Check sheet for the modelled part. Datum: model origin and axes. Units: mm. A direction names the side the tool comes from. Round coordinates to 2 decimals unless told otherwise and drop trailing zeros. Order: outer loops, then holes, each group sorted by start corner. A loop starts at its lowest first (then second) coordinate and runs counter-clockwise, first axis right, second up. Notation, with made-up numbers: (54, 35) -> (100, 35) arc R21 cw to (100, 48) -> close; hole circle Ø2 at (48.5, 12). An arc over 180 degrees is marked (long way). Answer in a Markdown table with one row per item.
Autodesk Inventor part; units mm, degrees
ref_plane "YZ Plane" through (0, 0, 0) normal (1, 0, 0) x (0, 1, 0)
ref_plane "XZ Plane" through (0, 0, 0) normal (0, 1, 0) x (-1, 0, 0)
ref_plane "XY Plane" through (0, 0, 0) normal (0, 0, 1) x (1, 0, 0)
sketch "Sketch1" plane through (0, 0, 0) normal (0, 0, 1) x (1, 0, 0)
  line L0 (0, 0) -> (6.15, 0)
  line L1 (6.15, 0) -> (6.15, 4.4)
  line L2 (6.15, 4.4) -> (0, 4.4)
  line L3 (0, 4.4) -> (0, 0)
  dimension "d0" = 6.15
  dimension "d1" = 4.4
extrude "Extrusion1" add sketch "Sketch1" against normal blind 4.7
sketch "Sketch2" plane through (0, 0, -4.7) normal (0, 0, -1) x (-1, 0, 0)
  line L0 (-6.15, 0) -> (-6.15, 4.4)
  line L1 (0, 4.4) -> (0, 0)
  line L2 (-6.15, 4.4) -> (0, 4.4)
  circle A0 centre (-4.545, 3.353) radius 0.25
  circle A1 centre (-1.605, 3.353) radius 0.25
  circle A2 centre (-4.545, 1.253) radius 0.25
  circle A3 centre (-1.605, 1.253) radius 0.25
  dimension "d4" = 0.5
  dimension "d5" = 0.5
  dimension "d6" = 0.5
  dimension "d7" = 0.5
  dimension "d8" = 3.44
  dimension "d9" = 3.44
  dimension "d10" = 2.6
  dimension "d11" = 2.6
  dimension "d12" = 1.605
  dimension "d13" = 1.605
  dimension "d14" = 1.605
  dimension "d15" = 1.047
extrude "Extrusion2" add sketch "Sketch2" along normal blind 25
properties part number "LineSensor"
Item 1: Cross-section at B-B (y = 2.55). Record the boundary of the cut face in (x, z).
Result sheet:
| item | result |
|---|---|
| outline | (0, -4.7) -> (6.15, -4.7) -> (6.15, 0) -> (0, 0) -> close |
Item 2: Cross-section at C-C (z = -17.5). Record the boundary of the cut face in (x, y) (3 decimals).
Result sheet:
| item | result |
|---|---|
| outline | circle Ø0.5 at (1.605, 1.253); circle Ø0.5 at (1.605, 3.353); circle Ø0.5 at (4.545, 1.253); circle Ø0.5 at (4.545, 3.353) |
Item 3: Cross-section at A-A (x = 2.25). Record the boundary of the cut face in (y, z).
Result sheet:
| item | result |
|---|---|
| outline | (0, -4.7) -> (4.4, -4.7) -> (4.4, 0) -> (0, 0) -> close |
Item 4: Scan lines: line 1 (X direction, y = 3.4, z = -25.75); line 2 (Z direction, x = 3, y = 2.7); line 3 (X direction, y = 3.15, z = -15.75). Record each from-to range of solid material in increasing order. Write a range as [from, to].
Result sheet:
| item | result |
|---|---|
| line 1 | x = [1.36, 1.85], [4.3, 4.79] |
| line 2 | z = [-4.7, 0] |
| line 3 | x = [1.46, 1.75], [4.4, 4.69] |
Item 5: Depth check by flat-ended pin: P1, Ø1.3, axis at x = 3.5, y = 3, coming from the -Z side; P2, Ø3, axis at x = 3.5, z = -7.5, coming from the +Y side; P3, Ø1, axis at x = 2.5, z = -6.5, coming from the +Y side. Enter the tip coordinate at first touch or a pass-through.
Result sheet:
| item | result |
|---|---|
| P1 | stops at z = -4.7 |
| P2 | stops at y = 3.6 |
| P3 | passes through |
Item 6: Set-up check for faces 1 (the flat face through (6.15, 2, -2)), 2 (the flat face through (3, 2, -4.7)): record each of +Z, -Z, +X, -X, +Y, -Y from which the full face is reachable in a straight line by a thin tool's end or side.
Result sheet:
| item | result |
|---|---|
| face 1 | +Z, -Z, +X, +Y, -Y |
| face 2 | -Z |
